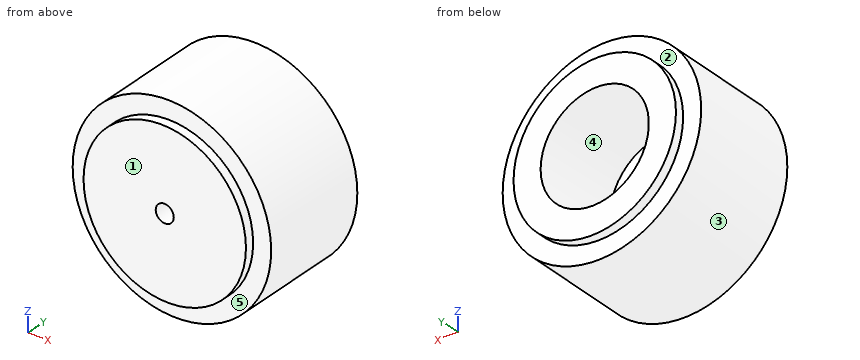
Autodesk Inventor part; units mm, degrees
ref_plane "YZ Plane" through (0, 0, 0) normal (1, 0, 0) x (0, 1, 0)
ref_plane "XZ Plane" through (0, 0, 0) normal (0, 1, 0) x (-1, 0, 0)
ref_plane "XY Plane" through (0, 0, 0) normal (0, 0, 1) x (1, 0, 0)
sketch "Náčrt1" plane through (0, 0, 0) normal (0, 1, 0) x (-1, 0, 0)
  circle A0 centre (0, 0) radius 16.5
  circle A1 centre (0, 0) radius 13.5
  dimension "d0" = 33
  dimension "d1" = 27
extrude "Vysunutí1" add sketch "Náčrt1" along normal mid plane 21 contours A1
sketch "Náčrt4" plane through (0, 0, 0) normal (1, 0, 0) x (0, 1, 0)
  line L0 (-10.5, 13.5) -> (-10.5, -13.5)
  point P0 (0, 0)
  point P1 (-6.5, 0)
  dimension "d16" = 4
hole "Díra2" at (0, -6.5, 0) direction (1, 0, 0) diameter 3 end through all
thread "Závit1"
extrude "Vysunutí2" add sketch "Náčrt1" along normal mid plane 18
sketch "Náčrt2" plane through (0, 10.5, 0) normal (0, 1, 0) x (1, 0, 0)
  circle A0 centre (0, 0) radius 9
  dimension "d6" = 18
extrude "Vysunutí3" cut sketch "Náčrt2" against normal blind 14.5
sketch "Náčrt3" plane through (0, -10.5, 0) normal (0, -1, 0) x (1, 0, 0)
  circle A0 centre (0, 0) radius 13.5
hole "Díra1" at (0, -10.5, 0) direction (0, 1, 0) diameter 3 end through all
properties part number "JSUMO_Wheel_33x20mm"
Verification items for the finished model (mm, model axes). Face numbers are marked on the shaded views. A direction names the side the tool comes from. Give positions to 0.01 mm unless a question says otherwise; leave off trailing zeros. Order: outer loops, then holes, each group sorted by start corner. A loop starts at its lowest first (then second) coordinate and runs counter-clockwise, first axis right, second up. Notation, with made-up numbers: (58, 39) - (76, 39) arc R13 ccw to (76, 44) - close; hole circle Ø8 at (4.25, 75.25). An arc over 180 degrees is marked (long way). Answer as CSV lines item,"result". Start each with the question number.
Item 1: Access from +Z, -Z, +X, -X, +Y, -Y to the whole of each face (thin tool, end or side, straight path). Record for the marked faces 1 and 2.
Item 2: Section check D-D, the plane x = 5.5. Record the boundary of the cut face in (y, z).
Item 3: Section check A-A, the plane z = 0. Record the boundary of the cut face in (x, y).
Item 4: Gauge pin test, flat ends, axial feed: pin 1 (8 mm diameter, centred on x = 11, y = 1, fed in from -Z); pin 2 (1.5 mm diameter, centred on x = -2, y = 8.5, fed in from -Z); pin 3 (8 mm diameter, centred on x = -7.5, y = 2.5, fed in from +Z). Record the tip position at first contact, or that the pin passes through.
Item 5: Section check C-C, the plane x = -6.5. Record the boundary of the cut face in (y, z).
Item 6: Section check B-B, the plane y = -6.5. Record the boundary of the cut face in (x, z), plus the area to 3 significant figures.
Item 7: Mould release check, pull along X, two halves, no side actions. Record for the marked faces 3, 4 and 5: released by +X, released by -X, zero draft, split by the parting line, or undercut.
Item 8: Material ranges on L1, parallel to Z at x = 0, y = 4.5; L2, parallel to Z at x = 6.25, y = -6.5; L3, parallel to Y at x = -14, z = -5, recorded low to high.
Filled in:
1,face 1,"+Z, -Z, +X, -X, -Y"
1,face 2,"+Y"
2,outline,"(-10.5, -12.33) - (-9, -12.33) - (-9, -15.56) - (9, -15.56) - (9, -12.33) - (10.5, -12.33) - (10.5, -7.12) - (-4, -7.12) - (-4, 7.12) - (10.5, 7.12) - (10.5, 12.33) - (9, 12.33) - (9, 15.56) - (-9, 15.56) - (-9, 12.33) - (-10.5, 12.33) - close; hole circle Ø3 at (-6.5, 0)"
3,outline,"(-16.5, -9) - (-13.5, -9) - (-13.5, -10.5) - (-1.5, -10.5) - (-1.5, -4) - (-9, -4) - (-9, 10.5) - (-13.5, 10.5) - (-13.5, 9) - (-16.5, 9) - close; (1.5, -10.5) - (13.5, -10.5) - (13.5, -9) - (16.5, -9) - (16.5, 9) - (13.5, 9) - (13.5, 10.5) - (9, 10.5) - (9, -4) - (1.5, -4) - (1.5, -5) - (13.5, -5) - (13.5, -8) - (1.5, -8) - close"
4,pin 1,"z = -14.94"
4,pin 2,"z = -16.45"
4,pin 3,"z = 16.12"
5,outline,"(-10.5, -11.83) - (-9, -11.83) - (-9, -15.17) - (9, -15.17) - (9, -11.83) - (10.5, -11.83) - (10.5, -6.22) - (-4, -6.22) - (-4, 6.22) - (10.5, 6.22) - (10.5, 11.83) - (9, 11.83) - (9, 15.17) - (-9, 15.17) - (-9, 11.83) - (-10.5, 11.83) - close"
6,outline,"circle Ø33 at (0, 0); hole (0, -1.5) - (13.42, -1.5) arc R13.5 ccw to (13.42, 1.5) - (0, 1.5) arc R1.5 ccw to start"
6,area,"811 mm^2"
7,face 3,"split by the parting line"
7,face 4,"undercut"
7,face 5,"zero draft"
8,L1,"-16.5 to -9, 9 to 16.5"
8,L2,"-15.27 to -1.5, 1.5 to 15.27"
8,L3,"-9 to 9"
